Here's how the part is built. I have some questions about the finished solid (model axes, mm). Face numbers are marked on the shaded views. A direction names the side the tool comes from. Coordinates: 2 decimals unless noted, no trailing zeros. Order: outer loops, then holes, each group sorted by start corner. A loop starts at its lowest first (then second) coordinate and runs counter-clockwise, first axis right, second up. Notation, with made-up numbers: (49.25, 68) - (71.25, 68) arc R17 cw to (71.25, 75) - close; hole circle Ø8 at (61, -8.5). An arc over 180 degrees is marked (long way). Use one line per item in the form item = value. Start each with the question number.
Autodesk Inventor part; units mm, degrees
ref_plane "YZ Plane" through (0, 0, 0) normal (1, 0, 0) x (0, 1, 0)
ref_plane "XZ Plane" through (0, 0, 0) normal (0, 1, 0) x (-1, 0, 0)
ref_plane "XY Plane" through (0, 0, 0) normal (0, 0, 1) x (1, 0, 0)
sketch "Sketch1" plane through (0, 0, 0) normal (0, 0, 1) x (1, 0, 0)
  line L0 (0, 0) -> (0, 3)
  line L1 (0, 3) -> (2, 3)
  line L2 (2, 3) -> (2, 2.5)
  line L3 (2, 2.5) -> (3, 2.5)
  line L4 (3, 2.5) -> (3, 3)
  line L5 (3, 3) -> (18, 3)
  line L6 (18, 3) -> (18, 5)
  line L7 (18, 5) -> (130, 5)
  line L8 (130, 5) -> (130, 0)
  line L9 (130, 0) -> (0, 0)
  line L10 (122, 5) -> (122, 0)
  dimension "d0" = 1
  dimension "d2" = 3
  dimension "d3" = 6
  dimension "d4" = 5
  dimension "d5" = 130
  dimension "d6" = 18
  dimension "d7" = 10
  dimension "d8" = 8
revolve "Revolution1" add sketch "Sketch1" angle 360 about axis through (130, 0, 0) along (-1, 0, 0)
thread "Thread1"
chamfer "Chamfer2" distance 0.5 angle 45 1 edges at (0, -3, 0)
sketch "Sketch2" plane through (0, 0, 0) normal (0, 1, 0) x (-1, 0, 0)
  circle A0 centre (-122, 0) radius 2.5
  point P0 (0, 0)
  dimension "d21" = 5
extrude "Extrusion1" cut sketch "Sketch2" along normal through all both and the other way through all
chamfer "Chamfer3" distance 1 angle 45 5 edges at (18, -5, 0) (130, -5, 0) (121.9995, 4.3301, -2.5) (122.0005, 4.3301, 2.5) (124.4999, -5, -0.0199)
properties part number "Rod" material "Stainless Steel"
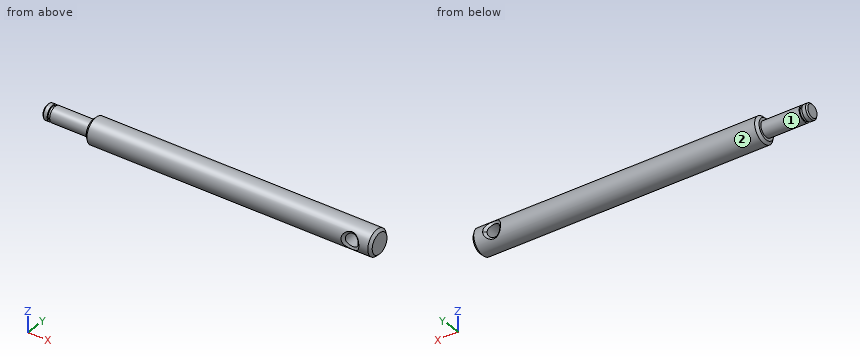
1) Suppose I cut it at B-B, the plane x = 117. List the corners of the cut face in (y, z) for me, then the cut area to 3 significant figures.
2) I need wall thicknesses on probe 1 along X at (y, z) = (2.25, 0); probe 2 along Z at (x, y) = (122, 0.5); probe 3 along Z at (x, y) = (47, 0.25). Which ranges of each line are inside material? Lowest first, please. Write a range as [from, to].
3) For pin 1 (3 mm diameter, centred on x = 67, z = 3.5, fed in from +Y); pin 2 (2 mm diameter, centred on y = 2.5, z = -3, fed in from -X); pin 3 (3 mm diameter, centred on x = 102.5, z = 3, fed in from +Y), each with a flat end and sliding along its axis, tell me the tip position at first contact or that it passes through.
4) Which directions (+Z, -Z, +X, -X, +Y, -Y) give clear straight access to the entire face, cutting with the end or side of a thin tool? Please do the marked faces 1 and 2.
5) Suppose I cut it at A-A, the plane y = 0. List the corners of the cut face in (x, z) for me, then the cut area to 3 significant figures.
From the geometry:
q1.outline = circle Ø10 at (0, 0)
q1.area = 78.5 mm2
q2.probe_1 = [0, 119.5], [124.5, 130]
q2.probe_2 = [-4.97, -2.5], [2.5, 4.97]
q2.probe_3 = [-4.99, 4.99]
q3.pin_1 = 4.58
q3.pin_2 = 0.41
q3.pin_3 = 4.77
q4.face_1 = -X
q4.face_2 = +X, -X
q5.outline = (0, -2.5) - (0.5, -3) - (2, -3) - (2, -2.5) - (3, -2.5) - (3, -3) - (18, -3) - (18, -4) - (19, -5) - (129, -5) - (130, -4) - (130, 4) - (129, 5) - (19, 5) - (18, 4) - (18, 3) - (3, 3) - (3, 2.5) - (2, 2.5) - (2, 3) - (0.5, 3) - (0, 2.5) - close; hole circle Ø5 at (122, 0)
q5.area = 1,210 mm2
